from build123d import *

# Parameters (mm, degrees)
F0_W     = 292.1
F0_H     = 31.75
F1_DEPTH = 20.32
F2_DEPTH = 5.08
F3_DEPTH = 25.4
F4_DEPTH = 25.4
F6_D     = 21
F6_DEPTH = 91
F6_TIP   = 6.3090364998


with BuildPart() as f1:
    # F0 (on Right) → F1 (new body)
    with BuildSketch(Plane.YZ):
        Rectangle(F0_W, F0_H)
    extrude(amount=F1_DEPTH)

    # F2 (add): a face of the model
    f2_faces = [f1.faces().sort_by_distance(p)[0] for p in [
        (20.32, 0, 0),
    ]]
    extrude(f2_faces, amount=F2_DEPTH)

    # F3 (add): a face of the model
    f3_faces = [f1.faces().sort_by_distance(p)[0] for p in [
        (25.4, 0, 0),
    ]]
    extrude(f3_faces, amount=F3_DEPTH)

    # F4 (cut): a face of the model
    f4_faces = [f1.faces().sort_by_distance(p)[0] for p in [
        (50.8, 0, 0),
    ]]
    extrude(f4_faces, amount=-F4_DEPTH, mode=Mode.SUBTRACT)

    # F6
    with Locations(Plane.XZ.offset(146.05)):
        with Locations((12.7, 0)):
            Hole(F6_D / 2, depth=F6_DEPTH)
            with Locations((0, 0, -(F6_DEPTH + F6_TIP / 2))):  # 118° drill point
                Cone(0, F6_D / 2, F6_TIP, mode=Mode.SUBTRACT)


solid = f1.part
CAD build for the part. Positions are in the model's coordinates, mm. A direction names the side the tool comes from. Round coordinates to 2 decimals unless told otherwise and drop trailing zeros. Write each loop counter-clockwise with the first axis right and the second up, starting at its lowest first coordinate (ties: lowest second). Pieces come first, ordered by that corner, then holes.
(1) 3-axis set-ups, long thin cutter, end or side, ignore diameter. For faces 1 (the face through (20.439, -99.913, 7.096)), 2 (the face through (13, -2, 15.875)): which of +Z, -Z, +X, -X, +Y, -Y reach the whole face in a straight line?
(2) Drop flat-ended pins along their axis: P1, Ø3, axis at x = 6.5, z = 1.5, coming from the -Y side; P2, Ø3, axis at x = 8.5, z = 7.5, coming from the -Y side. Give the stop position or say it passes through.
(3) Mould opens along X. For faces 3 (the face through (13, 146.05, 0)), 4 (the face through (0, -2, 0)), 5 (the face through (11.25, -49.84, -1.11)) say: pulls with the +X half, pulls with the -X half, needs draft (parallel to the pull), parting line crosses it, or undercut.
(4) Slice it at A-A, the plane y = -99. Write the cut outline in (x, z) (3 decimals).
(5) Probe line 1 along X through (y, z) = (-87, 0); line 2 along Z through (x, y) = (12.7, -101.5) (3 decimals); line 3 along X through (y, z) = (-62.5, -5). List the from-to ranges inside material, lowest first.
From the geometry:
1. face 1: -Y
1. face 2: +Z, +X, -X, +Y, -Y
2. P1: stops at y = -53.48
2. P2: stops at y = -54.81
3. face 3: needs draft
3. face 4: pulls with the -X half
3. face 5: undercut
4. outline: (0, -15.875) - (25.4, -15.875) - (25.4, 15.875) - (0, 15.875) - close; hole circle Ø21 at (12.7, 0)
5. line 1: x = 0 to 2.2, 23.2 to 25.4
5. line 2: z = -15.875 to -10.5, 10.5 to 15.875
5. line 3: x = 0 to 3.47, 21.93 to 25.4
